from build123d import *

# Parameters (mm, degrees)
SKETCH1_R           = 4.8
BOSS_EXTRUDE1_DEPTH = 9
SKETCH2_R           = 7.5
BOSS_EXTRUDE2_DEPTH = 2
CHAMFER1_SIZE       = 1


with BuildPart() as part:
    # Sketch1 → Boss-Extrude1 (new body)
    with BuildSketch(Plane(origin=(0, 0, 0), x_dir=(1, 0, 0), z_dir=(0, 1, 0))):
        with Locations(Location((0, 0, 0), (0, 0, 270))):
            Circle(SKETCH1_R)
    extrude(amount=BOSS_EXTRUDE1_DEPTH)

    # Sketch2 → Boss-Extrude2 (add)
    with BuildSketch(Plane.XZ):
        with Locations(Location((0, 0, 0), (0, 0, 270))):
            Circle(SKETCH2_R)
    extrude(amount=-BOSS_EXTRUDE2_DEPTH)

    # Chamfer1
    chamfer1_edges = [part.edges().sort_by_distance(p)[0] for p in [
        (0, 9, -4.8),
    ]]
    chamfer(chamfer1_edges, length=CHAMFER1_SIZE)


solid = part.part
Here's how the part is built. I have some questions about the finished solid (model axes, mm). A direction names the side the tool comes from. Coordinates: 2 decimals unless noted, no trailing zeros. Write each loop counter-clockwise with the first axis right and the second up, starting at its lowest first coordinate (ties: lowest second). Pieces come first, ordered by that corner, then holes.
Item 1: Will these pins go through, and if not, where does the flat tip stop? pin 1 (4 mm diameter, centred on y = 6.5, z = 1, fed in from +X); pin 2 (2 mm diameter, centred on x = 6, y = 7.5, fed in from -Z); pin 3 (4 mm diameter, centred on x = -3.5, y = 1.5, fed in from +Z); pin 4 (4 mm diameter, centred on y = 7, z = -4.5, fed in from -X).
Item 2: I want a section at A-A on x = 0. Write out the boundary of the cut face in (y, z), and give its area (3 significant figures).
Item 3: If I drill on line 1 (Y direction, x = -3.5, z = -3.75); line 2 (Z direction, x = 1.5, y = 6.5); line 3 (X direction, y = 6, z = 1), over which ranges is the centre line in solid material (lowest first)?
Item 4: I want a section at C-C on y = 3.75. Write out the boundary of the cut face in (x, z).
Item 5: I want a section at D-D on x = 5.75. Write out the boundary of the cut face in (y, z), and give its area (3 significant figures).
Item 6: On a 3-axis mill with a long thin cutter (end or side, diameter ignored), from which of +Z, -Z, +X, -X, +Y, -Y can I reach the whole of each face in a straight line? I mean faces 1 (the cylindrical face through (0.33, 0.986, 7.493)), 2 (the cylindrical face through (4.05, 4.96, 2.58)). Say none if no direction works.
Item 7: I want a section at B-B on z = 0. Write out the boundary of the cut face in (x, y).
Findings below:
1. pin 1: stops at x = 4.8
1. pin 2: passes through
1. pin 3: stops at z = 7.35
1. pin 4: stops at x = -4.1
2. outline: (0, -7.5) - (2, -7.5) - (2, -4.8) - (8, -4.8) - (9, -3.8) - (9, 3.8) - (8, 4.8) - (2, 4.8) - (2, 7.5) - (0, 7.5) - close
2. area: 96.2 mm2
3. line 1: y = 0 to 2
3. line 2: z = -4.56 to 4.56
3. line 3: x = -4.69 to 4.69
4. outline: circle Ø9.6 at (0, 0)
5. outline: (0, -4.82) - (2, -4.82) - (2, 4.82) - (0, 4.82) - close
5. area: 19.3 mm2
6. face 1: +Y, -Y
6. face 2: +Y
7. outline: (-7.5, 0) - (7.5, 0) - (7.5, 2) - (4.8, 2) - (4.8, 8) - (3.8, 9) - (-3.8, 9) - (-4.8, 8) - (-4.8, 2) - (-7.5, 2) - close
